```python
from build123d import *

# Parameters (mm, degrees)
SKETCH1_R           = 3.175
SKETCH1_R_2         = 1.5875
BOSS_EXTRUDE1_DEPTH = 25.4
CUT_EXTRUDE1_REACH  = 40.1
SKETCH2_W           = 12.7
SKETCH2_H           = 44.45


with BuildPart() as part:
    # Sketch1 → Boss-Extrude1 (new body)
    with BuildSketch(Plane.XY):
        with BuildLine():
            Line((-19.05, 50.8), (-19.05, -50.8))
            ThreePointArc((-19.05, -50.8), (0, -69.85), (19.05, -50.8))
            Line((19.05, -50.8), (19.05, 50.8))
            ThreePointArc((19.05, 50.8), (0, 69.85), (-19.05, 50.8))
        make_face()
        with Locations((0, 50.8)):
            Circle(SKETCH1_R, mode=Mode.SUBTRACT)
        with Locations((0, -50.8)):
            Circle(SKETCH1_R, mode=Mode.SUBTRACT)
        with Locations((0, 63.5)):
            Circle(SKETCH1_R_2, mode=Mode.SUBTRACT)
        with Locations((-12.7, 50.8)):
            Circle(SKETCH1_R_2, mode=Mode.SUBTRACT)
        with Locations((0, 38.1)):
            Circle(SKETCH1_R_2, mode=Mode.SUBTRACT)
        with Locations((12.7, 50.8)):
            Circle(SKETCH1_R_2, mode=Mode.SUBTRACT)
        with Locations((-12.7, -50.8)):
            Circle(SKETCH1_R_2, mode=Mode.SUBTRACT)
        with Locations((0, -38.1)):
            Circle(SKETCH1_R_2, mode=Mode.SUBTRACT)
        with Locations((12.7, -50.8)):
            Circle(SKETCH1_R_2, mode=Mode.SUBTRACT)
        with Locations((0, -63.5)):
            Circle(SKETCH1_R_2, mode=Mode.SUBTRACT)
    extrude(amount=BOSS_EXTRUDE1_DEPTH)

    # Sketch2 → Cut-Extrude1 (cut, up to next)
    with BuildSketch(Plane(origin=(19.05, 0, 0), x_dir=(0, 0, -1), z_dir=(1, 0, 0)), mode=Mode.PRIVATE) as cut_extrude1_sk1:
        with Locations((-6.35, 47.625)):
            Rectangle(SKETCH2_W, SKETCH2_H)
    cut_extrude1_tool1 = extrude(cut_extrude1_sk1.sketch, amount=-CUT_EXTRUDE1_REACH, mode=Mode.PRIVATE) & part.part
    add(cut_extrude1_tool1.solids().sort_by_distance((19.05, 47.625, 6.35))[0], mode=Mode.SUBTRACT)
    # Sketch2 → Cut-Extrude1 (cut, up to next)
    with BuildSketch(Plane(origin=(19.05, 0, 0), x_dir=(0, 0, -1), z_dir=(1, 0, 0)), mode=Mode.PRIVATE) as cut_extrude1_sk2:
        with Locations((-6.35, -47.625)):
            Rectangle(SKETCH2_W, SKETCH2_H)
    cut_extrude1_tool2 = extrude(cut_extrude1_sk2.sketch, amount=-CUT_EXTRUDE1_REACH, mode=Mode.PRIVATE) & part.part
    add(cut_extrude1_tool2.solids().sort_by_distance((19.05, -47.625, 6.35))[0], mode=Mode.SUBTRACT)


solid = part.part
```
Check sheet for the modelled part. Datum: model origin and axes. Units: mm. A direction names the side the tool comes from. Round coordinates to 2 decimals unless told otherwise and drop trailing zeros. Loops run counter-clockwise (first coordinate to the right, second up) from the corner with the lowest first, then second, coordinate; pieces in that order, holes last. Notation, with made-up numbers: M 88,35.5 L 137,35.5 A24 cw 137,55.5 Z; hole C 71,85.5 d1. An arc over 180 degrees is marked long. Answer as a JSON object with one key per item and string values.
1. Section check D-D (x = -5.5). Record the boundary of the cut face in (y, z), plus the area to 3 significant figures.
Reply:
{"outline": "M -69.04,12.7 L -25.4,12.7 L -25.4,0 L 25.4,0 L 25.4,12.7 L 69.04,12.7 L 69.04,25.4 L -69.04,25.4 Z", "area": "2,400 mm²"}
2. Access from +Z, -Z, +X, -X, +Y, -Y to the whole of each face (thin tool, end or side, straight path). Record for faces 5 (the cylindrical face through (-0.41, 53.95, 18.96)), 6 (the flat face through (0, 47, 12.7)), 7 (the flat face through (0, -25.4, 6)).
Reply:
{"face 5": "+Z, -Z", "face 6": "-Z, +X, -X, +Y", "face 7": "-Z, +X, -X, -Y"}
3. Mould release check, pull along X, two halves, no side actions. Record for faces 1 (the flat face through (0, 1, 25.4)), 2 (the cylindrical face through (0.419, 69.845, 18.961)), 3 (the cylindrical face through (-11.85, 52.14, 18.96)), 4 (the cylindrical face through (1.707, -48.123, 18.961)): pulls with the +X half, pulls with the -X half, needs draft (parallel to the pull), parting line crosses it, or undercut.
Reply:
{"face 1": "needs draft", "face 2": "parting line crosses it", "face 3": "undercut", "face 4": "undercut"}
4. Scan lines: line 1 (X direction, y = 38.1, z = 16.5); line 2 (Y direction, x = 12.7, z = 17.25); line 3 (Z direction, x = -5.5, y = 64). Record each from-to range of solid material in increasing order.
Reply:
{"line 1": "x = -19.05 to -1.59, 1.59 to 19.05", "line 2": "y = -65 to -52.39, -49.21 to 49.21, 52.39 to 65", "line 3": "z = 12.7 to 25.4"}
5. Section check B-B (z = 15.5). State how many separate pieces and enclosed holes the cut face has, plus the area to 3 significant figures.
Reply:
{"separate pieces": "1", "enclosed holes": "10", "area": "4,880 mm²"}
6. Section check C-C (x = -12.7). Record the boundary of the cut face in (y, z), plus the area to 3 significant figures.
Reply:
{"outline": "M -65,12.7 L -52.39,12.7 L -52.39,25.4 L -65,25.4 Z; M -49.21,12.7 L -25.4,12.7 L -25.4,0 L 25.4,0 L 25.4,12.7 L 49.21,12.7 L 49.21,25.4 L -49.21,25.4 Z; M 52.39,12.7 L 65,12.7 L 65,25.4 L 52.39,25.4 Z", "area": "2,220 mm²"}
7. Section check A-A (y = 38.1). Record the boundary of the cut face in (x, z).
Reply:
{"outline": "M -19.05,12.7 L -1.59,12.7 L -1.59,25.4 L -19.05,25.4 Z; M 1.59,12.7 L 19.05,12.7 L 19.05,25.4 L 1.59,25.4 Z"}
8. Gauge pin test, flat ends, axial feed: P1, Ø5, axis at x = -15, z = 11.5, coming from the +Y side; P2, Ø14, axis at x = -4.5, z = 6, coming from the +Y side; P3, Ø11.5, axis at x = 8, y = -42.5, coming from the -Z side. Record the tip position at first contact, or that the pin passes through.
Reply:
{"P1": "stops at y = 64.9", "P2": "stops at y = 69.69", "P3": "stops at z = 12.7"}
